Design review of the part built by this model. Coordinates are the model's own, in mm. Coordinates: 2 decimals unless noted, no trailing zeros. Write each loop counter-clockwise with the first axis right and the second up, starting at its lowest first coordinate (ties: lowest second). Pieces come first, ordered by that corner, then holes.
Q1. Clearance check with a flat-ended pin moving along its axis: pin 1 Ø5 at (x, z) = (-38, -18.5) entering from +Y. State where the tip first meets the part, or that it passes through.
Q2. The part is to be moulded in two halves that separate along Z. For faces 1 (the face through (-40.95, 2.54, -21.2)), 2 (the face through (103, 2, 1)), 3 (the face through (-1, 2, -60)), say which applies: +Z half, -Z half, draft (parallel to the pull), parting line (faces both ways), or undercut.
Q3. Add section A-A, the plane x = 81.5. Give the boundary of the cut face in (y, z), plus the area to 3 significant figures.
Q4. To check wall thickness, follow probe 1 along Z at (x, y) = (-38, 3.95); probe 2 along Z at (x, y) = (81.5, 2.9); probe 3 along X at (y, z) = (2.7, 20). State the ranges of each line that lie inside material, in increasing order.
from build123d import *

# Parameters (mm, degrees)
SKETCH_1_W          = 206
SKETCH_1_H          = 120
EXTRUDE_1_DEPTH     = 5
SKETCH_2_R          = 2.1
CUT_EXTRUDE_1_DEPTH = 6
SKETCH_3_R          = 4
CUT_EXTRUDE_2_DEPTH = 6


with BuildPart() as part:
    # 草图1 → 凸台-拉伸1 (new body)
    with BuildSketch(Plane(origin=(0, 0, 0), x_dir=(1, 0, 0), z_dir=(0, 1, 0))):
        Rectangle(SKETCH_1_W, SKETCH_1_H)
    extrude(amount=EXTRUDE_1_DEPTH)

    # 草图2 → 切除-拉伸1 (cut, through all)
    with BuildSketch(Plane(origin=(0, 5, 0), x_dir=(1, 0, 0), z_dir=(0, 1, 0))):
        with Locations((-81.5, 20)):
            Circle(SKETCH_2_R)
        with Locations((81.5, 20)):
            Circle(SKETCH_2_R)
        with Locations((81.5, -20)):
            Circle(SKETCH_2_R)
        with Locations((-81.5, -20)):
            Circle(SKETCH_2_R)
    extrude(amount=-CUT_EXTRUDE_1_DEPTH, mode=Mode.SUBTRACT)

    # 草图3 → 切除-拉伸2 (cut, through all)
    with BuildSketch(Plane(origin=(0, 5, 0), x_dir=(1, 0, 0), z_dir=(0, 1, 0))):
        with Locations((-38, 18.5)):
            Circle(SKETCH_3_R)
        with Locations((38, 18.5)):
            Circle(SKETCH_3_R)
        with Locations((38, -18.5)):
            Circle(SKETCH_3_R)
        with Locations((-38, -18.5)):
            Circle(SKETCH_3_R)
    extrude(amount=-CUT_EXTRUDE_2_DEPTH, mode=Mode.SUBTRACT)


solid = part.part
Here are the results:
1. pin 1: passes through
2. face 1: undercut
2. face 2: draft
2. face 3: -Z half
3. outline: (0, -60) - (5, -60) - (5, -22.1) - (0, -22.1) - close; (0, -17.9) - (5, -17.9) - (5, 17.9) - (0, 17.9) - close; (0, 22.1) - (5, 22.1) - (5, 60) - (0, 60) - close
3. area: 558 mm2
4. probe 1: z = -60 to -22.5, -14.5 to 14.5, 22.5 to 60
4. probe 2: z = -60 to -22.1, -17.9 to 17.9, 22.1 to 60
4. probe 3: x = -103 to -83.6, -79.4 to -41.71, -34.29 to 34.29, 41.71 to 79.4, 83.6 to 103
